Here's how the part is built. I have some questions about the finished solid (model axes, mm). A direction names the side the tool comes from. Round coordinates to 2 decimals unless told otherwise and drop trailing zeros. Write each loop counter-clockwise with the first axis right and the second up, starting at its lowest first coordinate (ties: lowest second). Pieces come first, ordered by that corner, then holes. Notation, with made-up numbers: (8, -7.5) -> (63, -7.5) arc R5 ccw to (63, 0.5) -> close; hole circle Ø6 at (-14.5, 62.25). An arc over 180 degrees is marked (long way). Answer in a Markdown table with one row per item. Add a question column.
from build123d import *

# Parameters (mm, degrees)
CROQUIS1_R                   = 23.75
CROQUIS1_R_2                 = 40
SALIENTE_EXTRUIR1_DEPTH      = 5.525
CROQUIS3_R                   = 23.75
SALIENTE_EXTRUIR3_DEPTH      = 4.7625
SALIENTE_EXTRUIR3_DEPTH_BACK = 4.7625
SALIENTE_EXTRUIR9_DEPTH      = 4.7625
SALIENTE_EXTRUIR9_DEPTH_BACK = 4.7625


with BuildPart() as part:
    # Croquis1 → Saliente-Extruir1 (new body)
    with BuildSketch(Plane.XY):
        Circle(CROQUIS1_R)
        with BuildLine():
            ThreePointArc((-3.25, 12.328828006), (0, -12.75), (3.25, 12.328828006))
            Line((3.25, 12.328828006), (3.25, 15.75))
            Line((3.25, 15.75), (-3.25, 15.75))
            Line((-3.25, 15.75), (-3.25, 12.328828006))
        make_face(mode=Mode.SUBTRACT)
        Circle(CROQUIS1_R_2)
        Circle(CROQUIS1_R, mode=Mode.SUBTRACT)
    extrude(amount=SALIENTE_EXTRUIR1_DEPTH)

    # Croquis3 → Saliente-Extruir3 (add, two sides)
    with BuildSketch(Plane.XY.offset(2.7625)) as saliente_extruir3_sk:
        Circle(CROQUIS3_R)
        with BuildLine():
            Line((-3.25, 15.75), (-3.25, 12.328828006))
            ThreePointArc((-3.25, 12.328828006), (0, -12.75), (3.25, 12.328828006))
            Line((3.25, 12.328828006), (3.25, 15.75))
            Line((3.25, 15.75), (-3.25, 15.75))
        make_face(mode=Mode.SUBTRACT)
    extrude(amount=SALIENTE_EXTRUIR3_DEPTH)
    extrude(saliente_extruir3_sk.sketch, amount=-SALIENTE_EXTRUIR3_DEPTH_BACK)

    # Croquis5 → Saliente-Extruir9 (add, two sides)
    with BuildSketch(Plane.XY.offset(2.7625)) as saliente_extruir9_sk:
        Polygon((11.452742746, -42.742217813), (25.5, -44.167295593), (22.125, -38.321624117), (36.062445841, -36.062445841), (31.289475068, -31.289475068), (44.167295593, -25.5), (38.321624117, -22.125), (49.262217141, -13.1997713), (42.742217813, -11.452742746), (51, 0), (44.25, 0), (49.262217141, 13.1997713), (42.742217813, 11.452742746), (44.167295593, 25.5), (38.321624117, 22.125), (36.062445841, 36.062445841), (31.289475068, 31.289475068), (25.5, 44.167295593), (22.125, 38.321624117), (13.1997713, 49.262217141), (11.452742746, 42.742217813), (0, 51), (0, 44.25), (-13.1997713, 49.262217141), (-11.452742746, 42.742217813), (-25.5, 44.167295593), (-22.125, 38.321624117), (-36.062445841, 36.062445841), (-31.289475068, 31.289475068), (-44.167295593, 25.5), (-38.321624117, 22.125), (-49.262217141, 13.1997713), (-42.742217813, 11.452742746), (-51, 0), (-44.25, 0), (-49.262217141, -13.1997713), (-42.742217813, -11.452742746), (-44.167295593, -25.5), (-38.321624117, -22.125), (-36.062445841, -36.062445841), (-31.289475068, -31.289475068), (-25.5, -44.167295593), (-22.125, -38.321624117), (-13.1997713, -49.262217141), (-11.452742746, -42.742217813), (0, -51), (0, -44.25), (13.1997713, -49.262217141), align=None)
        with BuildLine():
            Line((0, 38.2), (0, 40))
            ThreePointArc((0, 40), (5.180991094, 39.20639841), (9.886887523, 36.898366564))
            Line((9.886887523, 36.898366564), (10.352761804, 38.637033052))
            ThreePointArc((10.352761804, 38.637033052), (15.151815702, 36.529533612), (19.1, 33.082170425))
            Line((19.1, 33.082170425), (20, 34.641016151))
            ThreePointArc((20, 34.641016151), (24.090069109, 31.363241467), (27.011479041, 27.011479041))
            Line((27.011479041, 27.011479041), (28.284271247, 28.284271247))
            ThreePointArc((28.284271247, 28.284271247), (31.386624117, 24.059596246), (33.082170425, 19.1))
            Line((33.082170425, 19.1), (34.641016151, 20))
            ThreePointArc((34.641016151, 20), (36.544232561, 15.116329301), (36.898366564, 9.886887523))
            Line((36.898366564, 9.886887523), (38.637033052, 10.352761804))
            ThreePointArc((38.637033052, 10.352761804), (39.211411947, 5.142909495), (38.2, 0))
            Line((38.2, 0), (40, 0))
            ThreePointArc((40, 0), (39.20639841, -5.180991094), (36.898366564, -9.886887523))
            Line((36.898366564, -9.886887523), (38.637033052, -10.352761804))
            ThreePointArc((38.637033052, -10.352761804), (36.529533612, -15.151815702), (33.082170425, -19.1))
            Line((33.082170425, -19.1), (34.641016151, -20))
            ThreePointArc((34.641016151, -20), (31.363241467, -24.090069109), (27.011479041, -27.011479041))
            Line((27.011479041, -27.011479041), (28.284271247, -28.284271247))
            ThreePointArc((28.284271247, -28.284271247), (24.059596246, -31.386624117), (19.1, -33.082170425))
            Line((19.1, -33.082170425), (20, -34.641016151))
            ThreePointArc((20, -34.641016151), (15.116329301, -36.544232561), (9.886887523, -36.898366564))
            Line((9.886887523, -36.898366564), (10.352761804, -38.637033052))
            ThreePointArc((10.352761804, -38.637033052), (5.142909495, -39.211411947), (0, -38.2))
            Line((0, -38.2), (0, -40))
            ThreePointArc((0, -40), (-5.180991094, -39.20639841), (-9.886887523, -36.898366564))
            Line((-9.886887523, -36.898366564), (-10.352761804, -38.637033052))
            ThreePointArc((-10.352761804, -38.637033052), (-15.151815702, -36.529533612), (-19.1, -33.082170425))
            Line((-19.1, -33.082170425), (-20, -34.641016151))
            ThreePointArc((-20, -34.641016151), (-24.090069109, -31.363241467), (-27.011479041, -27.011479041))
            Line((-27.011479041, -27.011479041), (-28.284271247, -28.284271247))
            ThreePointArc((-28.284271247, -28.284271247), (-31.386624117, -24.059596246), (-33.082170425, -19.1))
            Line((-33.082170425, -19.1), (-34.641016151, -20))
            ThreePointArc((-34.641016151, -20), (-36.544232561, -15.116329301), (-36.898366564, -9.886887523))
            Line((-36.898366564, -9.886887523), (-38.637033052, -10.352761804))
            ThreePointArc((-38.637033052, -10.352761804), (-39.211411947, -5.142909495), (-38.2, 0))
            Line((-38.2, 0), (-40, 0))
            ThreePointArc((-40, 0), (-39.20639841, 5.180991094), (-36.898366564, 9.886887523))
            Line((-36.898366564, 9.886887523), (-38.637033052, 10.352761804))
            ThreePointArc((-38.637033052, 10.352761804), (-36.529533612, 15.151815702), (-33.082170425, 19.1))
            Line((-33.082170425, 19.1), (-34.641016151, 20))
            ThreePointArc((-34.641016151, 20), (-31.363241467, 24.090069109), (-27.011479041, 27.011479041))
            Line((-27.011479041, 27.011479041), (-28.284271247, 28.284271247))
            ThreePointArc((-28.284271247, 28.284271247), (-24.059596246, 31.386624117), (-19.1, 33.082170425))
            Line((-19.1, 33.082170425), (-20, 34.641016151))
            ThreePointArc((-20, 34.641016151), (-15.116329301, 36.544232561), (-9.886887523, 36.898366564))
            Line((-9.886887523, 36.898366564), (-10.352761804, 38.637033052))
            ThreePointArc((-10.352761804, 38.637033052), (-5.142909495, 39.211411947), (0, 38.2))
        make_face(mode=Mode.SUBTRACT)
    extrude(amount=SALIENTE_EXTRUIR9_DEPTH)
    extrude(saliente_extruir9_sk.sketch, amount=-SALIENTE_EXTRUIR9_DEPTH_BACK)


solid = part.part
Item 1: On a 3-axis mill with a long thin cutter (end or side, diameter ignored), from which of +Z, -Z, +X, -X, +Y, -Y can I reach the whole of each face in a straight line? I mean faces 4 (the flat face through (46.72, 6.51, 2.83)), 5 (the cylindrical face through (-36.528, -15.188, -0.986)), 6 (the cylindrical face through (-5.149, -23.185, 6.511)). Say none if no direction works.
Item 2: I need wall thicknesses on line 1 along Y through (x, z) = (-35.5, 5.75); line 2 along X through (y, z) = (3.5, -1.5); line 3 along Z through (x, y) = (-11, 26) (3 decimals). Which ranges of each line are inside material? Lowest first, please. Write a range as from..to.
Item 3: If we section it at A-A on x = -1.5: Please give me the cut outline in (y, z) (3 decimals).
Item 4: If we mould it in two halves opening along Y, with no side actions, what happens to faces 1 (the flat face through (-17.72, -43.72, 2.83)), 2 (the cylindrical face through (-31.352, -24.125, -0.986)), 3 (the flat face through (12.34, 46.05, 2.83))? For each: pulls with the +Y half, pulls with the -Y half, needs draft (parallel to the pull), parting line crosses it, or undercut.
Item 5: If we section it at C-C on y = 7.5: Please give me the cut outline in (x, z) (3 decimals).
Item 6: If we section it at B-B on y = -41.5: Please give me the cut outline in (x, z) (3 decimals), then the cut area to 3 significant figures.
Item 7: For P1, Ø0.9, axis at x = -38.5, z = 6.5, coming from the +Y side; P2, Ø1.5, axis at x = -29, z = 0.5, coming from the +Y side; P3, Ø3.5, axis at y = 49, z = 2.5, coming from the -X side, each with a flat end and sliding along its axis, tell me the tip position at first contact or that it passes through.
Results list:
| question | item | result |
|---|---|---|
| 1 | face 4 | +Z, -Z, +X |
| 1 | face 5 | -Z |
| 1 | face 6 | +Z |
| 2 | line 1 | -35.5..-18.3, 16.6..29.4, 35.5..36.15 |
| 2 | line 2 | -48.48..-39.64, -23.49..-12.26, 12.26..23.49, 39.06..45.58 |
| 2 | line 3 | 0..5.525 |
| 3 | outline | (-49.918, -2) -> (-39.935, -2) -> (-39.935, 0) -> (-23.703, 0) -> (-23.703, -2) -> (-12.661, -2) -> (-12.661, 7.525) -> (-23.703, 7.525) -> (-23.703, 5.525) -> (-39.935, 5.525) -> (-39.935, 7.525) -> (-49.918, 7.525) -> close; (15.75, -2) -> (23.703, -2) -> (23.703, 0) -> (38.665, 0) -> (38.665, -2) -> (44.82, -2) -> (44.82, 7.525) -> (38.665, 7.525) -> (38.665, 5.525) -> (23.703, 5.525) -> (23.703, 7.525) -> (15.75, 7.525) -> close |
| 4 | face 1 | pulls with the -Y half |
| 4 | face 2 | undercut |
| 4 | face 3 | pulls with the +Y half |
| 5 | outline | (-45.592, -2) -> (-38.291, -2) -> (-38.291, 0) -> (-22.535, 0) -> (-22.535, -2) -> (-10.311, -2) -> (-10.311, 7.525) -> (-22.535, 7.525) -> (-22.535, 5.525) -> (-38.291, 5.525) -> (-38.291, 7.525) -> (-45.592, 7.525) -> close; (10.311, -2) -> (22.535, -2) -> (22.535, 0) -> (39.15, 0) -> (39.15, -2) -> (47.098, -2) -> (47.098, 7.525) -> (39.15, 7.525) -> (39.15, 5.525) -> (22.535, 5.525) -> (22.535, 7.525) -> (10.311, 7.525) -> close |
| 6 | outline | (-26.699, -2) -> (-23.96, -2) -> (-23.96, 7.525) -> (-26.699, 7.525) -> close; (-19.532, -2) -> (23.96, -2) -> (23.96, 7.525) -> (-19.532, 7.525) -> close |
| 6 | area | 440 mm² |
| 7 | P1 | y = 28.25 |
| 7 | P2 | y = 37.33 |
| 7 | P3 | x = -13.2 |
